The listing builds one solid part. Answer for the finished solid, in the listing's coordinates (mm). A direction names the side the tool comes from. Give positions to 0.01 mm unless a question says otherwise; leave off trailing zeros. Loops run counter-clockwise (first coordinate to the right, second up) from the corner with the lowest first, then second, coordinate; pieces in that order, holes last. Notation, with made-up numbers: (0.5, 24) - (48.5, 24) arc R29 cw to (48.5, 55) - close; hole circle Ø6 at (48.25, 32.25). An arc over 180 degrees is marked (long way). Write each question's results on one line, items separated by ' | '.
from build123d import *

# Parameters (mm, degrees)
COVERBASEEXTRUDE_DEPTH      = 304.8
COVERBASEEXTRUDE_DEPTH_BACK = 304.8
COVERSHELL_T                = -2


with BuildPart() as part:
    # Sketch1 → CoverBaseExtrude (new, two sides: drawn at the far end of the back side and taken through both)
    with BuildSketch(Plane(origin=(0, 0, 0), x_dir=(0, 0, -1), z_dir=(1, 0, 0)).offset(-COVERBASEEXTRUDE_DEPTH_BACK)):
        with BuildLine():
            Line((-152.4, 0), (152.4, 0))
            ThreePointArc((152.4, 0), (183.830896424, 13.019103576), (196.85, 44.45))
            Line((196.85, 44.45), (-196.85, 44.45))
            ThreePointArc((-196.85, 44.45), (-183.830896424, 13.019103576), (-152.4, 0))
        make_face()
    extrude(amount=COVERBASEEXTRUDE_DEPTH + COVERBASEEXTRUDE_DEPTH_BACK)

    # CoverShell
    covershell_openings = [part.faces().sort_by_distance(p)[0] for p in [
        (0, 44.45, 0),
    ]]
    offset(amount=COVERSHELL_T, openings=covershell_openings, kind=Kind.INTERSECTION)


solid = part.part
Item 1: A cutting plane is placed at B-B, the plane y = 16. Determine the outline of the cut face in (x, z).
Values found:
outline: (-304.8, -186.55) - (304.8, -186.55) - (304.8, 186.55) - (-304.8, 186.55) - close; hole (-302.8, -183.91) - (302.8, -183.91) - (302.8, 183.91) - (-302.8, 183.91) - close
Item 2: Find the intervals of material crossed by line 1 along X through (y, z) = (10, -62.5); line 2 along Z through (x, y) = (111.5, 34.5); line 3 along Y through (x, z) = (-235.5, 59), in increasing order. Write a range as [from, to].
Values found:
line 1: x = [-304.8, -302.8], [302.8, 304.8] | line 2: z = [-195.72, -193.67], [193.67, 195.72] | line 3: y = [0, 2]
Item 3: For faces 4 (the face through (-4.239, 14.105, -182.085)), 5 (the face through (304.8, 23, 3)), determine the directions among +Z, -Z, +X, -X, +Y, -Y from which every point of the face is accessible in a straight line to the end or side of a thin tool.
Values found:
face 4: +Y | face 5: +Z, -Z, +X, +Y, -Y
Item 4: For a pull along Z with two mould halves and no side action, classify faces 1 (the face through (-304.8, 23, 3)), 2 (the face through (-4.239, 14.765, 182.745)), 3 (the face through (-4.267, 13.367, 184.175)) as released by +Z, released by -Z, zero draft, split by the parting line, or undercut.
Values found:
face 1: zero draft | face 2: undercut | face 3: released by +Z
Item 5: A cutting plane is placed at A-A, the plane x = -16. Determine the outline of the cut face in (y, z), plus the area to 3 significant figures.
Values found:
outline: (0, -152.4) arc R44.45 ccw to (44.45, -196.85) - (44.45, -194.85) arc R42.45 cw to (2, -152.4) - (2, 152.4) arc R42.45 cw to (44.45, 194.85) - (44.45, 196.85) arc R44.45 ccw to (0, 152.4) - close | area: 883 mm²
Item 6: A cutting plane is placed at C-C, the plane z = 80.5. Determine the outline of the cut face in (x, y), plus the area to 3 significant figures.
Values found:
outline: (-304.8, 0) - (304.8, 0) - (304.8, 44.45) - (302.8, 44.45) - (302.8, 2) - (-302.8, 2) - (-302.8, 44.45) - (-304.8, 44.45) - close | area: 1,390 mm²
Item 7: Flat-ended cylindrical pins translate along their axes: P1, Ø6, axis at x = 35, y = 30.5, coming from the -Z side; P2, Ø1.5, axis at x = 5.5, y = 23.5, coming from the +Z side (3 decimals); P3, Ø3, axis at x = 46.5, z = 18.5, coming from the +Y side. Find the tip coordinate at first contact, or state that the pin passes through.
Values found:
P1: stops at z = -195.48 | P2: stops at z = 191.995 | P3: stops at y = 2
